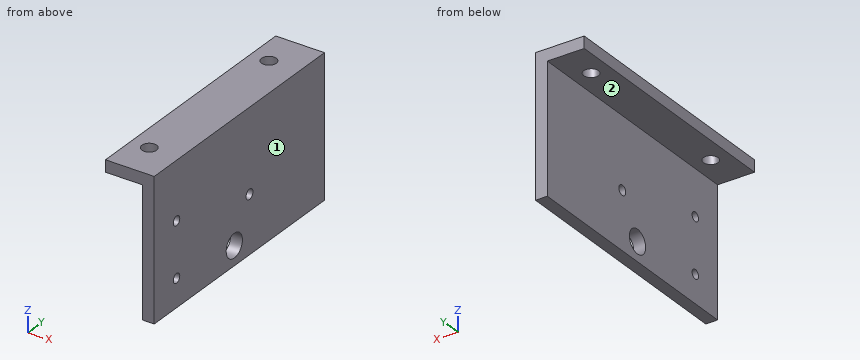
Solid Edge part; units mm, degrees
sketch "Sketch1" plane through (0, 0, 0) normal (1, 0, 0) x (0, 1, 0)
  line L0 (0, 0) -> (168, 0)
  line L1 (168, 95) -> (168, 0)
  line L2 (168, 95) -> (0, 95)
  line L3 (0, 95) -> (0, 0)
  dimension "D1" = 168
extrude "Protrusion1" add sketch "Sketch1" against normal blind 8
hole "Hole_1" at (0, 79, 13) direction (-1, 0, 0) diameter 16 end through all
sketch "Sketch2" plane through (0, 76.5, 47.5) normal (1, 0, 0) x (0, 1, 0)
  circle A0 centre (17.5, -8.5192) radius 3
extrude "Cutout1" cut sketch "Sketch2" against normal blind 50.8
hole "Hole_2" at (0, 94, 38.9808) direction (-1, 0, 0) diameter 6.8 end through all
sketch "Sketch3" plane through (-8, 84, 47.5) normal (-1, 0, 0) x (0, 1, 0)
  line L0 (-84, -39.5) -> (84, -39.5)
  line L1 (84, -39.5) -> (84, -47.5)
  line L2 (84, -47.5) -> (-84, -47.5)
  line L3 (-84, -47.5) -> (-84, -39.5)
  dimension "D1" = 84
extrude "ExtrudedProtrusion_2" add sketch "Sketch3" along normal blind 25
hole "Hole_3" at (-20.5, 143, 87) direction (0, 0, 1) diameter 10 end up to next
hole "Hole1" at (-20.5, 25, 87) direction (0, 0, 1) diameter 10 end up to next
hole "Hole_7" at (-8, 22, 56) direction (1, 0, 0) diameter 6.35 end up to next
hole "Hole2" at (-8, 22, 19) direction (1, 0, 0) diameter 6.35 end up to next
properties part number "88866"
Design review of the part built by this model. Coordinates are the model's own, in mm. Face numbers are marked on the shaded views. A direction names the side the tool comes from. Give positions to 0.01 mm unless a question says otherwise; leave off trailing zeros. Write each loop counter-clockwise with the first axis right and the second up, starting at its lowest first coordinate (ties: lowest second). Pieces come first, ordered by that corner, then holes. Notation, with made-up numbers: M 46,81.25 L 99,81.25 A20 ccw 99,105.25 Z; hole C -4,-12 d11. An arc over 180 degrees is marked long. Answer as a JSON object with one key per item and string values. Group by question number.
1) For line 1 along Z through (x, y) = (-4.5, 22) (3 decimals); line 2 along Y through (x, z) = (-20.5, 90); line 3 along Z through (x, y) = (-2, 79), list the stretches that pass through material, from the lowest coordinate up.
2) We need section B-B (z = 55). Give the boundary of the cut face in (x, y).
3) Tool access review of the marked faces 1 and 2: name each direction out of +Z, -Z, +X, -X, +Y, -Y from which nothing blocks a thin tool from reaching the whole face with its end or side.
4) We need section D-D (y = 79). Give the boundary of the cut face in (x, z).
5) We need section C-C (x = -20.5). Give the boundary of the cut face in (y, z), and give its area (3 significant figures).
6) Clearance check with flat-ended pins moving along their axes: pin 1 Ø10 at (y, z) = (22, 56) entering from -X; pin 2 Ø12.5 at (x, y) = (-26.5, 59.5) entering from -Z. State where each tip first meets the part, or that it passes through.
7) We need section A-A (y = 143). Give the boundary of the cut face in (x, z).
Answer key:
{
 "1": {"line 1": "z = 0 to 15.825, 22.175 to 52.825, 59.175 to 95", "line 2": "y = 0 to 20, 30 to 138, 148 to 168", "line 3": "z = 0 to 5, 21 to 95"},
 "2": {"outline": "M -8,0 L 0,0 L 0,18.99 L -8,18.99 Z; M -8,25.01 L 0,25.01 L 0,168 L -8,168 Z"},
 "3": {"face 1": "+Z, -Z, +X, +Y, -Y", "face 2": "-Z, -X, +Y, -Y"},
 "4": {"outline": "M -33,87 L -8,87 L -8,21 L 0,21 L 0,95 L -33,95 Z; M -8,0 L 0,0 L 0,5 L -8,5 Z"},
 "5": {"outline": "M 0,87 L 20,87 L 20,95 L 0,95 Z; M 30,87 L 138,87 L 138,95 L 30,95 Z; M 148,87 L 168,87 L 168,95 L 148,95 Z", "area": "1,180 mm²"},
 "6": {"pin 1": "stops at x = -8", "pin 2": "stops at z = 87"},
 "7": {"outline": "M -33,87 L -25.5,87 L -25.5,95 L -33,95 Z; M -15.5,87 L -8,87 L -8,0 L 0,0 L 0,95 L -15.5,95 Z"}
}
